Input: part model. Units: mm. Frame: model coordinates. Coordinates: 2 decimals unless noted, no trailing zeros. Order: outer loops, then holes, each group sorted by start corner. A loop starts at its lowest first (then second) coordinate and runs counter-clockwise, first axis right, second up.
Autodesk Inventor part; units mm, degrees
ref_plane "YZ Plane" through (0, 0, 0) normal (1, 0, 0) x (0, 1, 0)
ref_plane "XZ Plane" through (0, 0, 0) normal (0, 1, 0) x (-1, 0, 0)
ref_plane "XY Plane" through (0, 0, 0) normal (0, 0, 1) x (1, 0, 0)
ref_plane "Work Plane1" through (0, 0, 0) normal (0, 0, 1) x (1, 0, 0)
sketch "Sketch1" plane through (0, 0, 0) normal (0, 0, 1) x (1, 0, 0)
  circle A0 centre (-2.8988, -0.3038) radius 16.3 construction
  circle A1 centre (-2.8988, -0.3038) radius 15.6
  circle A2 centre (-2.8988, -0.3038) radius 17
  line L0 (12.6983, 0) -> (14.0985, 0)
  line L1 (12.1151, 3.932) -> (13.4417, 4.3855)
  point P0 (0, 0)
  dimension "d0" = 0.7
  dimension "d1" = 0.7
  dimension "d4" = 34
extrude "Extrusion1" add sketch "Sketch1" along normal blind 2 contours A1 L0 A2 L1 picked at (13.4719, -1.6516)
properties part number "11_Lens_Thorlabs_Mount_Ring_B"
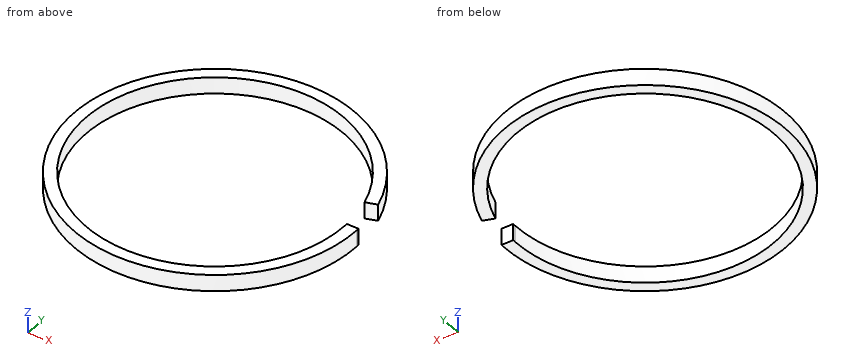
Item 1: Ray query, probe 1 along Y at (x, z) = (-4, 0.85); probe 2 along Y at (x, z) = (-8.5, 0.6); probe 3 along X at (y, z) = (-1, 0.8). Return the intervals inside material, ascending.
Response values:
probe 1: y = -17.27 to -15.86, 15.26 to 16.66
probe 2: y = -16.35 to -14.86, 14.26 to 15.75
probe 3: x = -19.88 to -18.48, 12.69 to 14.09
Item 2: Cut plane C-C on z = 1.35. Return loops of the section in (x, y), then the cut area to 3 significant figures.
Response values:
outline: (12.12, 3.93) - (13.44, 4.39) arc R17 ccw (long way) to (14.1, 0) - (12.7, 0) arc R15.6 cw (long way) to start
area: 137 mm2
Item 3: Pin query (flat end, axial travel): pin 1 Ø1.1 at (x, z) = (13, 0.5) entering from +Y. Return the tip coordinate at first contact, or that it passes through.
Response values:
pin 1: stops at y = 7
Item 4: Cut plane A-A on y = -4.5. Return loops of the section in (x, z).
Response values:
outline: (-19.37, 0) - (-17.92, 0) - (-17.92, 2) - (-19.37, 2) - close; (12.13, 0) - (13.58, 0) - (13.58, 2) - (12.13, 2) - close
Item 5: Cut plane B-B on x = 1.5. Return loops of the section in (y, z).
Response values:
outline: (-16.72, 0) - (-15.27, 0) - (-15.27, 2) - (-16.72, 2) - close; (14.66, 0) - (16.12, 0) - (16.12, 2) - (14.66, 2) - close
Item 6: Cut plane D-D on y = 3. Return loops of the section in (x, z).
Response values:
outline: (-19.57, 0) - (-18.14, 0) - (-18.14, 2) - (-19.57, 2) - close
